Autodesk Fusion 360 part; units mm, degrees
sketch "Esboço1" plane through (0, 0, 0) normal (0, 1, 0) x (1, 0, 0)
  circle A0 centre (0, 0) radius 8
  circle A1 centre (0, 0) radius 4
  dimension "d1" = 16
  dimension "d2" = 8
extrude "Extrusão1" add sketch "Esboço1" along normal blind 3.9
sketch "Esboço2" plane through (0, 3.9, 0) normal (0, 1, 0) x (-1, 0, 0)
  circle A0 centre (0, 0) radius 4
  circle A1 centre (0, 0) radius 8
  circle A2 centre (0, 0) radius 9
  dimension "d5" = 18
extrude "Extrusão2" add sketch "Esboço2" along normal blind 1.1 contours A1 | A2
chamfer "Chanfro1" distance 0.3 angle 45 1 edges at (-7.4586, 0, 2.8929)
chamfer "Chanfro2" distance 0.3 angle 45 1 edges at (8.3909, 3.9, -3.2545)
The listing builds one solid part. Answer for the finished solid, in the listing's coordinates (mm). A direction names the side the tool comes from. Round coordinates to 2 decimals unless told otherwise and drop trailing zeros. Write each loop counter-clockwise with the first axis right and the second up, starting at its lowest first coordinate (ties: lowest second). Pieces come first, ordered by that corner, then holes. Notation, with made-up numbers: (4, 7) -> (49, 7) arc R16 ccw to (49, 26) -> close; hole circle Ø10 at (81.25, -1.75). An arc over 180 degrees is marked (long way). Answer as a JSON object with one key per item and string values. Group by question number.
Q1. Each of these flat-tipped pins is pushed along its axis until it touches: pin 1 Ø3 at (y, z) = (2, -0.5) entering from +X; pin 2 Ø3 at (x, y) = (6.5, 1) entering from +Z (3 decimals); pin 3 Ø1 at (x, y) = (5, 3) entering from -Z. Where does it stop, or does it pass through?
Q2. Straight lines are drawn through the part: line 1 along X through (y, z) = (3.8, 0); line 2 along X through (y, z) = (0.2, 0). For each, find the intervals that lie inside material, in ascending order.
Q3. Which of the six approach directions +Z, -Z, +X, -X, +Y, -Y give full straight-line access (tool end or side, diameter ignored) to faces 1 (the face through (-1.73, 2.07, -7.81)), 2 (the face through (-2, 5, -4))?
Q4. Section A-A (y = 4.65) is taken. Write down the section's boundary in (x, z).
Q5. Section C-C (y = 2.2) is taken. Write down the section's boundary in (x, z).
Check values:
{
 "1": {"pin 1": "x = 8", "pin 2": "z = 6.245", "pin 3": "z = -6.61"},
 "2": {"line 1": "-8 to -4, 4 to 8", "line 2": "-7.9 to -4, 4 to 7.9"},
 "3": {"face 1": "-Y", "face 2": "+Z, -Z, +X, -X, +Y"},
 "4": {"outline": "circle Ø18 at (0, 0); hole circle Ø8 at (0, 0)"},
 "5": {"outline": "circle Ø16 at (0, 0); hole circle Ø8 at (0, 0)"}
}
